from build123d import *

# Parameters (mm, degrees)
SKETCH1_W           = 60
SKETCH1_H           = 60
BOSS_EXTRUDE1_DEPTH = 15
SKETCH2_W           = 30
SKETCH2_H           = 30
BOSS_EXTRUDE2_DEPTH = 20
SKETCH3_R           = 10
BOSS_EXTRUDE3_DEPTH = 15
SKETCH4_R           = 6
CUT_EXTRUDE1_DEPTH  = 66.574385243
CHAMFER1_SIZE       = 10
FILLET1_R           = 2
SHELL1_OUTLINE_R    = 9
SHELL1_DEPTH        = 12
SHELL1_START        = 12
SHELL1_2_OUTLINE_W  = 24
SHELL1_2_OUTLINE_H  = 24
SHELL1_2_OUTLINE_R  = 9
SHELL1_2_DEPTH      = 20


# Read off the part's stored shape, not the designer's step: Shell1
with BuildPart() as part:
    # Sketch1 → Boss-Extrude1 (new body)
    with BuildSketch(Plane.XY):
        Rectangle(SKETCH1_W, SKETCH1_H)
    extrude(amount=BOSS_EXTRUDE1_DEPTH)

    # Sketch2 → Boss-Extrude2 (add)
    with BuildSketch(Plane.XY.offset(15)):
        Rectangle(SKETCH2_W, SKETCH2_H)
    extrude(amount=BOSS_EXTRUDE2_DEPTH)

    # Sketch3 → Boss-Extrude3 (add)
    with BuildSketch(Plane.XY.offset(35)):
        Circle(SKETCH3_R)
    extrude(amount=BOSS_EXTRUDE3_DEPTH)

    # Sketch4 → Cut-Extrude1 (cut, through all)
    with BuildSketch(Plane.XY.offset(50)):
        Circle(SKETCH4_R)
    extrude(amount=-CUT_EXTRUDE1_DEPTH, mode=Mode.SUBTRACT)

    # Chamfer1
    chamfer1_edges = [part.edges().sort_by_distance(p)[0] for p in [
        (30, -30, 7.5),
        (-30, -30, 7.5),
        (-30, 30, 7.5),
        (30, 30, 7.5),
    ]]
    chamfer(chamfer1_edges, length=CHAMFER1_SIZE)

    # Fillet1
    fillet1_edges = [part.edges().sort_by_distance(p)[0] for p in [
        (15, -15, 25),
        (15, 15, 25),
        (-15, 15, 25),
        (-15, -15, 25),
    ]]
    fillet(fillet1_edges, radius=FILLET1_R)

    # Shell1 outline → Shell1 (cut)
    with BuildSketch(Plane.XY):
        Polygon((27, -18.757359313), (27, 18.757359313), (18.757359313, 27), (-18.757359313, 27), (-27, 18.757359313), (-27, -18.757359313), (-18.757359313, -27), (18.757359313, -27), align=None)
        Circle(SHELL1_OUTLINE_R, mode=Mode.SUBTRACT)
    extrude(amount=SHELL1_DEPTH, mode=Mode.SUBTRACT)

    # Shell1 2 outline → Shell1 2 (cut)
    with BuildSketch(Plane.XY.offset(SHELL1_START)):
        Rectangle(SHELL1_2_OUTLINE_W, SHELL1_2_OUTLINE_H)
        Circle(SHELL1_2_OUTLINE_R, mode=Mode.SUBTRACT)
    extrude(amount=SHELL1_2_DEPTH, mode=Mode.SUBTRACT)


solid = part.part
Read the model definition and answer for the solid it produces. Units are mm, in the model's axes. A direction names the side the tool comes from. Round coordinates to 2 decimals unless told otherwise and drop trailing zeros. Write each loop counter-clockwise with the first axis right and the second up, starting at its lowest first coordinate (ties: lowest second). Pieces come first, ordered by that corner, then holes.
Q1. Straight lines are drawn through the part: line 1 (Y direction, x = 0, z = 28); line 2 (X direction, y = 12.5, z = 11). For each, find the intervals that lie inside material, in ascending order.
Values:
line 1: y = -15 to -12, -9 to -6, 6 to 9, 12 to 15
line 2: x = -30 to -27, 27 to 30
Q2. A tool of negligible diameter and unlimited length cuts with its end or side. For faces 5 (the face through (-0.2, 10.2, 35)), 6 (the face through (-27, 0, 6)), 7 (the face through (-14.4, -14.43, 25.14)), 8 (the face through (15, 0, 25)), from which of +Z, -Z, +X, -X, +Y, -Y can it reach the whole face along a straight path? Write none if from no direction.
Values:
face 5: +Z
face 6: -Z
face 7: +Z, -X, -Y
face 8: +Z, +X, +Y, -Y
Q3. Find section D-D on x = -17. Determine the outline of the cut face in (y, z).
Values:
outline: (-30, 0) - (-27, 0) - (-27, 12) - (27, 12) - (27, 0) - (30, 0) - (30, 15) - (-30, 15) - close
Q4. Flat-ended cylindrical pins translate along their axes: P1, Ø5, axis at y = 8.5, z = 31, coming from the -X side; P2, Ø6, axis at x = 10, z = 24, coming from the -Y side; P3, Ø4, axis at y = -7, z = 25, coming from the +X side. Find the tip coordinate at first contact, or state that the pin passes through.
Values:
P1: stops at x = -15
P2: stops at y = -15
P3: stops at x = 15
Q5. The mould has two halves that part along Y. Classify faces 1 (the face through (-15, 0, 25)), 2 (the face through (0, 12, 22)), 3 (the face through (5, 8, 32)), 4 (the face through (-25, -25, 7)): released by +Y, released by -Y, zero draft, split by the parting line, or undercut.
Values:
face 1: zero draft
face 2: undercut
face 3: undercut
face 4: released by -Y
Q6. Find section C-C on z = 29.5. Determine the outline of the cut face in (x, y), and give its area (3 significant figures).
Values:
outline: (-15, -13) arc R2 ccw to (-13, -15) - (13, -15) arc R2 ccw to (15, -13) - (15, 13) arc R2 ccw to (13, 15) - (-13, 15) arc R2 ccw to (-15, 13) - close; circle Ø18 at (0, 0); hole (-12, -12) - (12, -12) - (12, 12) - (-12, 12) - close; hole circle Ø12 at (0, 0)
area: 462 mm2
Q7. Find section A-A on y = 0. Determine the outline of the cut face in (x, z).
Values:
outline: (-30, 0) - (-27, 0) - (-27, 12) - (-12, 12) - (-12, 32) - (-9, 32) - (-9, 0) - (-6, 0) - (-6, 50) - (-10, 50) - (-10, 35) - (-15, 35) - (-15, 15) - (-30, 15) - close; (6, 0) - (9, 0) - (9, 32) - (12, 32) - (12, 12) - (27, 12) - (27, 0) - (30, 0) - (30, 15) - (15, 15) - (15, 35) - (10, 35) - (10, 50) - (6, 50) - close
